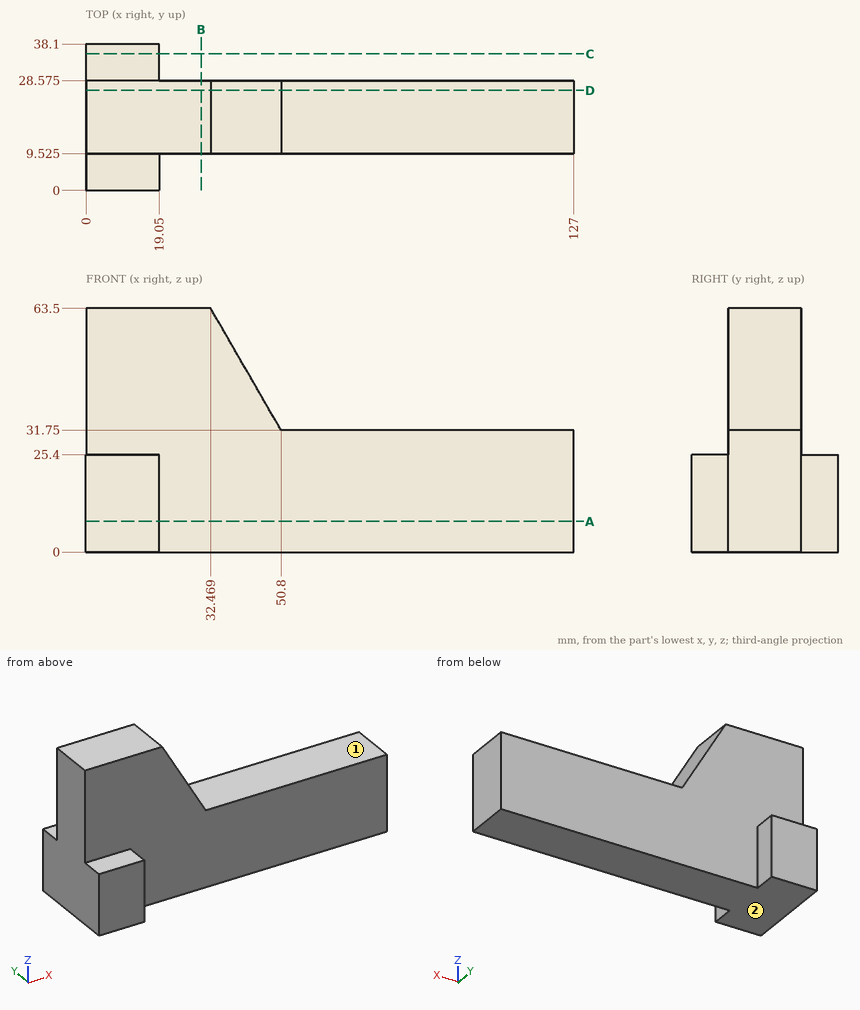
Check sheet for the drawn part. Datum: minimum x, y, z corner. Units: mm. A direction names the side the tool comes from. Coordinates: 2 decimals unless noted, no trailing zeros. Loops run counter-clockwise (first coordinate to the right, second up) from the corner with the lowest first, then second, coordinate; pieces in that order, holes last. Notation, with made-up numbers: (80.25, 19.5) -> (130.25, 19.5) arc R12 cw to (130.25, 39.5) -> close; hole circle Ø7 at (75.25, 64). An arc over 180 degrees is marked (long way). Answer as CSV lines item,"result".
1) Cross-section at B-B, the plane x = 30. Record the cut outline in (y, z) (3 decimals), then the cut area to 3 significant figures.
Found:
outline,"(9.525, 0) -> (28.575, 0) -> (28.575, 63.5) -> (9.525, 63.5) -> close"
area,"1,210 mm2"
2) Thickness scan on L1, parallel to Y at x = 103, z = 5 (3 decimals); L2, parallel to Z at x = 111.5, y = 25.5; L3, parallel to X at y = 29, z = 24. Record the ranges inside material, lowest first. Write a range as from..to.
Found:
L1,"y = 9.525..28.575"
L2,"z = 0..31.75"
L3,"x = 0..19.05"
3) Cross-section at A-A, the plane z = 8. Record the cut outline in (x, y) (3 decimals), then the cut area to 3 significant figures.
Found:
outline,"(0, 0) -> (19.05, 0) -> (19.05, 9.525) -> (127, 9.525) -> (127, 28.575) -> (19.05, 28.575) -> (19.05, 38.1) -> (0, 38.1) -> close"
area,"2,780 mm2"
4) Cross-section at D-D, the plane y = 26. Record the cut outline in (x, z).
Found:
outline,"(0, 0) -> (127, 0) -> (127, 31.75) -> (50.8, 31.75) -> (32.47, 63.5) -> (0, 63.5) -> close"
5) Cross-section at C-C, the plane y = 35.5. Record the cut outline in (x, z), then the cut area to 3 significant figures.
Found:
outline,"(0, 0) -> (19.05, 0) -> (19.05, 25.4) -> (0, 25.4) -> close"
area,"484 mm2"
6) Depth check by flat-ended pin: pin 1 (21 mm diameter, centred on x = 87.5, y = 19.5, fed in from +Z); pin 2 (19 mm diameter, centred on x = 56.5, z = 23.5, fed in from -Y) (3 decimals); pin 3 (1 mm diameter, centred on y = 7.5, z = 52.5, fed in from +X); pin 4 (3 mm diameter, centred on x = 11, y = 7, fed in from +Z). Enter the tip coordinate at first touch or a pass-through.
Found:
pin 1,"stops at z = 31.75"
pin 2,"stops at y = 9.525"
pin 3,"passes through"
pin 4,"stops at z = 25.4"
7) Tool access check on the marked faces 1 and 2. Record the directions out of +Z, -Z, +X, -X, +Y, -Y that give a thin tool (end or side, any length) a straight path to the whole face; none if there is none.
Found:
face 1,"+Z, +X, +Y, -Y"
face 2,"-Z, +X, -X, +Y, -Y"
